from build123d import *

# Parameters (mm, degrees)
SKETCH1_W           = 77
SKETCH1_H           = 60
SKETCH1_R           = 1.75
BOSS_EXTRUDE1_DEPTH = 3.5
SKETCH2_W           = 77
SKETCH2_H           = 5
BOSS_EXTRUDE2_DEPTH = 30
CUT_EXTRUDE1_DEPTH  = 20
SKETCH4_R           = 2
CUT_EXTRUDE2_DEPTH  = 20
RIB2_REACH          = 95.823
SKETCH5_WALL_W      = 232.071524048
SKETCH5_WALL_H      = 6
CHAMFER1_SIZE       = 20
FILLET1_R           = 10


with BuildPart() as part:
    # Sketch1 → Boss-Extrude1 (new body)
    with BuildSketch(Plane.XY):
        with Locations((-12, 11.85)):
            Rectangle(SKETCH1_W, SKETCH1_H)
        with Locations((-24, 35.8)):
            Circle(SKETCH1_R, mode=Mode.SUBTRACT)
        with Locations((-24, 0)):
            Circle(SKETCH1_R, mode=Mode.SUBTRACT)
        Circle(SKETCH1_R, mode=Mode.SUBTRACT)
    extrude(amount=BOSS_EXTRUDE1_DEPTH)

    # Sketch2 → Boss-Extrude2 (add)
    with BuildSketch(Plane.XY.offset(3.5)):
        with Locations((-12, 14.35)):
            Rectangle(SKETCH2_W, SKETCH2_H)
    extrude(amount=BOSS_EXTRUDE2_DEPTH)

    # Sketch3 → Cut-Extrude1 (cut)
    with BuildSketch(Plane(origin=(0, 16.85, 0), x_dir=(1, 0, 0), z_dir=(0, 1, 0))):
        with BuildLine():
            Line((-17.875, -18.5), (-17.875, -33.5))
            Line((-17.875, -33.5), (-6.125, -33.5))
            Line((-6.125, -33.5), (-6.125, -18.5))
            ThreePointArc((-6.125, -18.5), (-12, -12.625), (-17.875, -18.5))
        make_face()
    extrude(amount=-CUT_EXTRUDE1_DEPTH, mode=Mode.SUBTRACT)

    # Sketch4 → Cut-Extrude2 (cut)
    with BuildSketch(Plane(origin=(0, 16.85, 0), x_dir=(1, 0, 0), z_dir=(0, 1, 0))):
        with Locations(Location((13, -18.5, 0), (0, 0, 270))):
            Circle(SKETCH4_R)
        with Locations(Location((-37, -18.5, 0), (0, 0, 270))):
            Circle(SKETCH4_R)
    extrude(amount=-CUT_EXTRUDE2_DEPTH, mode=Mode.SUBTRACT)

    # Sketch5 wall → Rib2 (add, up to next)
    with BuildSketch(Plane(origin=(26.5, -3.15, 18.5), x_dir=(0, -0.707106781187, -0.707106781187), z_dir=(0, 0.707106781187, -0.707106781187)), mode=Mode.PRIVATE) as rib2_sk1:
        with Locations((0, 3)):
            Rectangle(SKETCH5_WALL_W, SKETCH5_WALL_H)
    rib2_tool1 = extrude(rib2_sk1.sketch, amount=RIB2_REACH, mode=Mode.PRIVATE) - part.part
    rib2 = rib2_tool1.solids().sort_by_distance((26.5, -3.15, 18.5))[0]
    add(rib2)

    # Mirror1: Rib2 across plane
    add(rib2.mirror(Plane(origin=(-12, 0, 0), x_dir=(0, 0, 1), z_dir=(1, 0, 0))))

    # Chamfer1
    chamfer1_edges = [part.edges().sort_by_distance(p)[0] for p in [
        (-50.5, 41.85, 1.75),
        (26.5, 41.85, 1.75),
    ]]
    chamfer(chamfer1_edges, length=CHAMFER1_SIZE)

    # Fillet1
    fillet1_edges = [part.edges().sort_by_distance(p)[0] for p in [
        (-50.5, 21.85, 1.75),
        (-30.5, 41.85, 1.75),
        (26.5, 21.85, 1.75),
        (6.5, 41.85, 1.75),
    ]]
    fillet(fillet1_edges, radius=FILLET1_R)


solid = part.part
Build history of the part. All positions in model axes, mm. A direction names the side the tool comes from. Give positions to 0.01 mm unless a question says otherwise; leave off trailing zeros. Loops run counter-clockwise (first coordinate to the right, second up) from the corner with the lowest first, then second, coordinate; pieces in that order, holes last. Notation, with made-up numbers: (1.5, 59.25) - (38.5, 59.25) arc R17 cw to (38.5, 69.25) - close; hole circle Ø9 at (-3, -13). An arc over 180 degrees is marked (long way). Write item = value, one per line. Start each with the question number.
1) Band-saw the part on C-C on z = 29.5. Give the cut face in (x, y) (3 decimals), plus the area to 3 significant figures.
2) Band-saw the part on B-B on y = 0. Give the cut face in (x, z).
3) Tool access for faces 4 (the flat face through (-6.125, 14, 26)), 5 (the flat face through (-12, -3, 3.5)), 6 (the flat face through (-13, 27, 3.5)): list every direction of +Z, -Z, +X, -X, +Y, -Y with a clear straight run to the whole face (end or side of a thin tool).
4) Band-saw the part on D-D on x = -24. Give the cut face in (y, z), plus the area to 4 significant figures.
5) Pull direction Z, two halves, no side cores. Call faces 1 (the flat face through (23.46, -2.94, 18.71)), 2 (the cylindrical face through (14.352, 14.385, 17.026)), 3 (the cylindrical face through (-49.76, 21.48, 1.77)): +Z half, -Z half, draft (parallel to the pull), parting line (faces both ways), or undercut.
6) Drop flat-ended pins along their axis: pin 1 Ø5 at (x, z) = (6, 9) entering from -Y; pin 2 Ø15 at (x, y) = (-21.5, -10.5) entering from +Z; pin 3 Ø3 at (x, y) = (0, 0) entering from +Z; pin 4 Ø5 at (x, z) = (-37, 18.5) entering from +Y. Give the stop position or say it passes through.
7) Probe probe 1 along X at (y, z) = (13.75, 18.5) (3 decimals); probe 2 along Y at (x, z) = (-24, 2.8); probe 3 along X at (y, z) = (-0.5, 14). List the from-to ranges inside material, lowest first. Write a range as from..to.
8) Band-saw the part on A-A on x = -37. Give the cut face in (y, z), plus the area to 3 significant figures.
Final values:
q1.outline = (-50.5, 7.85) - (-44.5, 7.85) - (-44.5, 11.85) - (-17.875, 11.85) - (-17.875, 16.85) - (-50.5, 16.85) - close; (-6.125, 11.85) - (20.5, 11.85) - (20.5, 7.85) - (26.5, 7.85) - (26.5, 16.85) - (-6.125, 16.85) - close
q1.area = 374 mm²
q2.outline = (-50.5, 0) - (-25.75, 0) - (-25.75, 3.5) - (-44.5, 3.5) - (-44.5, 21.65) - (-50.5, 21.65) - close; (-22.25, 0) - (-1.75, 0) - (-1.75, 3.5) - (-22.25, 3.5) - close; (1.75, 0) - (26.5, 0) - (26.5, 21.65) - (20.5, 21.65) - (20.5, 3.5) - (1.75, 3.5) - close
q3.face_4 = +Z, +Y, -Y
q3.face_5 = +Z, -Y
q3.face_6 = +Z, +X, -X, +Y
q4.outline = (-18.15, 0) - (-1.75, 0) - (-1.75, 3.5) - (-18.15, 3.5) - close; (1.75, 0) - (34.05, 0) - (34.05, 3.5) - (16.85, 3.5) - (16.85, 33.5) - (11.85, 33.5) - (11.85, 3.5) - (1.75, 3.5) - close; (37.55, 0) - (41.85, 0) - (41.85, 3.5) - (37.55, 3.5) - close
q4.area = 335.5 mm²
q5.face_1 = +Z half
q5.face_2 = undercut
q5.face_3 = draft
q6.pin_1 = 11.85
q6.pin_2 = 3.5
q6.pin_3 = through
q6.pin_4 = 16.85
q7.probe_1 = -50.5..-39, -35..-17.875, -6.125..11, 15..26.5
q7.probe_2 = -18.15..-1.75, 1.75..34.05, 37.55..41.85
q7.probe_3 = -50.5..-44.5, 20.5..26.5
q8.outline = (-18.15, 0) - (35.35, 0) - (35.35, 3.5) - (16.85, 3.5) - (16.85, 16.5) - (11.85, 16.5) - (11.85, 3.5) - (-18.15, 3.5) - close; (11.85, 20.5) - (16.85, 20.5) - (16.85, 33.5) - (11.85, 33.5) - close
q8.area = 317 mm²
